The drawing under review shows one solid part. Ordinate dimensions are in mm from its lowest x, y, z. A direction names the side the tool comes from. Give positions to 0.01 mm unless a question says otherwise; leave off trailing zeros. Write each loop counter-clockwise with the first axis right and the second up, starting at its lowest first coordinate (ties: lowest second). Pieces come first, ordered by that corner, then holes.
Q1. Mouldability with a two-part tool opening along Y and no side actions: class the marked faces 1, 2 and 3 as released by +Y, released by -Y, zero draft, split by the parting line, or undercut.
Q2. We need section D-D (y = 59). Write out the cut boundary in (x, z).
Q3. Machinability: for the marked faces 4, 5 and 6, which of the approach directions +Z, -Z, +X, -X, +Y, -Y give a long, thin tool a straight path to every point of the face, cutting with its end or side? Answer none if there is none.
Q4. We need section B-B (y = 37.5). Write out the cut boundary in (x, z), then the cut area to 3 significant figures.
Q5. We need section A-A (x = 38). Write out the cut boundary in (y, z), then the cut area to 3 significant figures.
Q6. We need section C-C (z = 14.5). Write out the cut boundary in (x, y).
Q7. For line 1 (X direction, y = 10, z = 7); line 2 (X direction, y = 40, z = 16); line 3 (Y direction, x = 13, z = 9.5), list the stretches that pass through material, from the lowest coordinate up.
Q8. Insertion check: P1, Ø0.7, axis at x = 1, y = 34, coming from the +Z side; P2, Ø8, axis at y = 20, z = 5.5, coming from the -X side; P3, Ø18.5, axis at x = 15, z = 24, coming from the -Y side (1 decimal). Each pin has a flat end and moves straight along its axis. Give the tip position at first contact, or say it passes through.
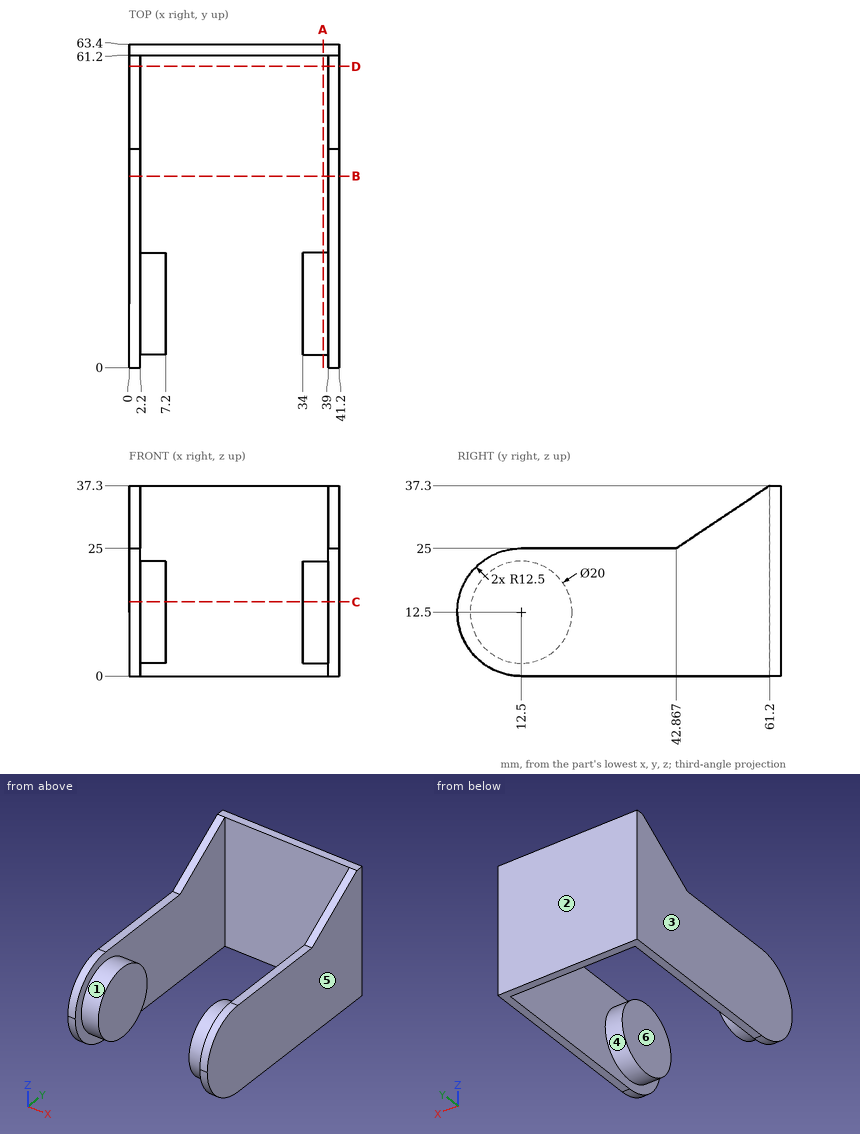
Computed:
1. face 1: undercut
1. face 2: released by +Y
1. face 3: zero draft
2. outline: (0, 0) - (2.2, 0) - (2.2, 35.82) - (0, 35.82) - close; (39, 0) - (41.2, 0) - (41.2, 35.82) - (39, 35.82) - close
3. face 4: none
3. face 5: +Z, -Z, +X, +Y, -Y
3. face 6: +Z, -Z, -Y
4. outline: (0, 0) - (2.2, 0) - (2.2, 25) - (0, 25) - close; (39, 0) - (41.2, 0) - (41.2, 25) - (39, 25) - close
4. area: 110 mm2
5. outline: circle Ø20 at (12.5, 12.5); (61.2, 0) - (63.4, 0) - (63.4, 37.3) - (61.2, 37.3) - close
5. area: 396 mm2
6. outline: (0, 0.16) - (2.2, 0.16) - (2.2, 2.7) - (7.2, 2.7) - (7.2, 22.3) - (2.2, 22.3) - (2.2, 61.2) - (39, 61.2) - (39, 22.3) - (34, 22.3) - (34, 2.7) - (39, 2.7) - (39, 0.16) - (41.2, 0.16) - (41.2, 63.4) - (0, 63.4) - close
7. line 1: x = 0 to 7.2, 34 to 41.2
7. line 2: x = 0 to 2.2, 39 to 41.2
7. line 3: y = 61.2 to 63.4
8. P1: stops at z = 25
8. P2: stops at x = 0
8. P3: stops at y = 4.9
